from build123d import *

# Parameters (mm, degrees)
SKETCH1_R           = 1.5
BOSS_EXTRUDE1_DEPTH = 8.4


with BuildPart() as part:
    # Sketch1 → Boss-Extrude1 (new body)
    with BuildSketch(Plane(origin=(0, 0, 0), x_dir=(1, 0, 0), z_dir=(0, 1, 0))):
        with BuildLine():
            Line((-160, 25), (-59.260530911, 25))
            ThreePointArc((-59.260530911, 25), (-57, 17.7), (-54.739469089, 25))
            Line((-54.739469089, 25), (77.739469089, 25))
            ThreePointArc((77.739469089, 25), (80, 17.7), (82.260530911, 25))
            Line((82.260530911, 25), (160, 25))
            Line((160, 25), (160, 13.2))
            Line((160, 13.2), (155, 13.2))
            Line((155, 13.2), (155, 14.7))
            Line((155, 14.7), (152, 14.7))
            Line((152, 14.7), (152, 13.2))
            Line((152, 13.2), (150.5, 13.2))
            Line((150.5, 13.2), (150.5, 9.2))
            Line((150.5, 9.2), (152, 9.2))
            Line((152, 9.2), (152, 7.7))
            Line((152, 7.7), (155, 7.7))
            Line((155, 7.7), (155, 9.2))
            Line((155, 9.2), (160, 9.2))
            Line((160, 9.2), (160, 0))
            Line((160, 0), (168, 0))
            Line((168, 0), (168, -8))
            Line((168, -8), (160, -8))
            Line((160, -8), (160, -12.4))
            Line((160, -12.4), (155, -12.4))
            Line((155, -12.4), (155, -10.9))
            Line((155, -10.9), (152, -10.9))
            Line((152, -10.9), (152, -12.4))
            Line((152, -12.4), (150.5, -12.4))
            Line((150.5, -12.4), (150.5, -16.4))
            Line((150.5, -16.4), (152, -16.4))
            Line((152, -16.4), (152, -17.9))
            Line((152, -17.9), (155, -17.9))
            Line((155, -17.9), (155, -16.4))
            Line((155, -16.4), (160, -16.4))
            Line((160, -16.4), (160, -25))
            Line((160, -25), (-160, -25))
            Line((-160, -25), (-160, -16.4))
            Line((-160, -16.4), (-155, -16.4))
            Line((-155, -16.4), (-155, -17.9))
            Line((-155, -17.9), (-152, -17.9))
            Line((-152, -17.9), (-152, -16.4))
            Line((-152, -16.4), (-150.5, -16.4))
            Line((-150.5, -16.4), (-150.5, -12.4))
            Line((-150.5, -12.4), (-152, -12.4))
            Line((-152, -12.4), (-152, -10.9))
            Line((-152, -10.9), (-155, -10.9))
            Line((-155, -10.9), (-155, -12.4))
            Line((-155, -12.4), (-160, -12.4))
            Line((-160, -12.4), (-160, -8))
            Line((-160, -8), (-168, -8))
            Line((-168, -8), (-168, 0))
            Line((-168, 0), (-160, 0))
            Line((-160, 0), (-160, 9.2))
            Line((-160, 9.2), (-155, 9.2))
            Line((-155, 9.2), (-155, 7.7))
            Line((-155, 7.7), (-152, 7.7))
            Line((-152, 7.7), (-152, 9.2))
            Line((-152, 9.2), (-150.5, 9.2))
            Line((-150.5, 9.2), (-150.5, 13.2))
            Line((-150.5, 13.2), (-152, 13.2))
            Line((-152, 13.2), (-152, 14.7))
            Line((-152, 14.7), (-155, 14.7))
            Line((-155, 14.7), (-155, 13.2))
            Line((-155, 13.2), (-160, 13.2))
            Line((-160, 13.2), (-160, 25))
        make_face()
        with Locations((11.5, 20.3)):
            Circle(SKETCH1_R, mode=Mode.SUBTRACT)
        with Locations((11.5, 10.3)):
            Circle(SKETCH1_R, mode=Mode.SUBTRACT)
        with Locations((87.1, 21.7)):
            Circle(SKETCH1_R, mode=Mode.SUBTRACT)
        with Locations((72.9, 21.7)):
            Circle(SKETCH1_R, mode=Mode.SUBTRACT)
        with Locations((-49.9, 21.7)):
            Circle(SKETCH1_R, mode=Mode.SUBTRACT)
        with Locations((-64.1, 21.7)):
            Circle(SKETCH1_R, mode=Mode.SUBTRACT)
    extrude(amount=BOSS_EXTRUDE1_DEPTH)


solid = part.part
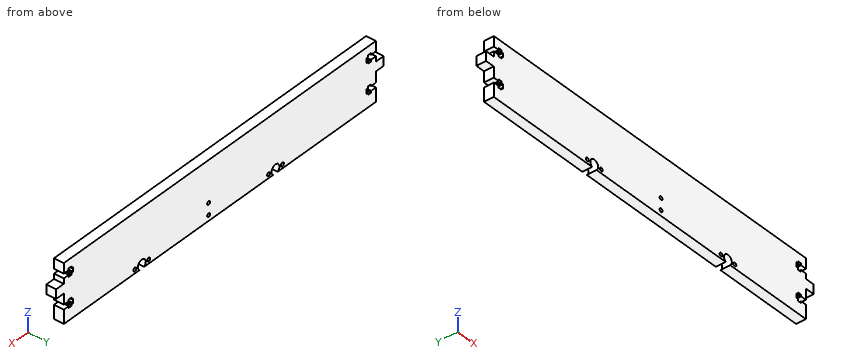
Geometry check sheet. Reference: the model listing, model coordinates, mm. Coordinates: 2 decimals unless noted, no trailing zeros. Answer in a Markdown table with one row per item. Add a question column.
1) Cross-section at A-A, the plane y = 5.75. State how many separate pieces and enclosed holes the cut face has, then the cut area to 3 significant figures.
2) Material ranges on line 1 along X through (y, z) = (5, -8); line 2 along Z through (x, y) = (11.5, 2.5); line 3 along Z through (x, y) = (-152.5, 3.5), recorded low to high. Write a range as [from, to].
3) Gauge pin test, flat ends, axial feed: P1, Ø2.5, axis at y = 5, z = -6.5, coming from the +X side; P2, Ø3.5, axis at y = 5, z = 11, coming from the -X side. Record the tip position at first contact, or that the pin passes through.
Check result:
| question | item | result |
|---|---|---|
| 1 | separate pieces | 1 |
| 1 | enclosed holes | 6 |
| 1 | area | 15,800 mm² |
| 2 | line 1 | x = [-160, -155], [-152, 152], [155, 160] |
| 2 | line 2 | z = [-25, -21.8], [-18.8, -11.8], [-8.8, 25] |
| 2 | line 3 | z = [-25, -14.7], [-7.7, 10.9], [17.9, 25] |
| 3 | P1 | stops at x = 160 |
| 3 | P2 | stops at x = -160 |
